Can you work these out from the model? Positions are in its coordinate system, mm. Face numbers are marked on the shaded views. A direction names the side the tool comes from. Coordinates: 2 decimals unless noted, no trailing zeros. Loops run counter-clockwise (first coordinate to the right, second up) from the corner with the lowest first, then second, coordinate; pieces in that order, holes last. Notation, with made-up numbers: M 23.5,20.25 L 54.5,20.25 A29 cw 54.5,46.25 Z; hole C -28,75 d10. An arc over 180 degrees is marked long. Answer as a JSON object with one key per item and string values. Group by question number.
Item 1: Suppose I cut it at A-A (z = -14). Write out the boundary of the cut face in (x, y).
Item 2: Which directions (+Z, -Z, +X, -X, +Y, -Y) give clear straight access to the entire face, cutting with the end or side of a thin tool? Please do the marked faces 1, 2 and 3.
Item 3: If I drill on line 1 (Z direction, x = 0, y = -2.75); line 2 (Y direction, x = 4.25, z = -21); line 3 (X direction, y = -2.5, z = -1.5), over which ranges is the centre line in solid material (lowest first)?
Item 4: Suppose I cut it at C-C (z = -26). Write out the boundary of the cut face in (x, y), then the cut area to 3 significant figures.
Item 5: We'd pull the mould along Z, two halves only. Please class the marked faces 4, 5 and 6: +Z half, -Z half, draft (parallel to the pull), parting line (faces both ways), or undercut.
Item 6: I'm going to push flat-ended pins straight in: pin 1 Ø5.5 at (x, z) = (2, -16) entering from -Y; pin 2 Ø6 at (x, z) = (0.5, -1) entering from -Y; pin 3 Ø1.5 at (x, y) = (-4.5, -2.5) entering from +Z; pin 4 Ø6 at (x, z) = (0, 0) entering from +Y. Where does each tip first touch, or does it pass through?
Item 7: Suppose I cut it at B-B (x = 0). Count the separate pieces of the cut face and the enclosed holes in it, then the cut area to 3 significant figures.
```python
from build123d import *

# Parameters (mm, degrees)
SKETCH1_R           = 0.75
BOSS_EXTRUDE1_DEPTH = 2.25
CUT_EXTRUDE1_DEPTH  = 7
SKETCH3_W           = 6
SKETCH3_H           = 3.5
CUT_EXTRUDE2_DEPTH  = 1
DRAFT1_ANGLE        = 30
DRAFT2_ANGLE        = 30
SKETCH4_R           = 3.9
CUT_EXTRUDE3_DEPTH  = 2
SKETCH5_R           = 4.8
BOSS_EXTRUDE2_DEPTH = 2
CHAMFER1_SIZE       = 1
SKETCH6_R           = 3
CUT_EXTRUDE4_DEPTH  = 3.5
SKETCH7_R           = 1.5
CUT_EXTRUDE5_DEPTH  = 4


with BuildPart() as part:
    # Sketch1 → Boss-Extrude1 (new body, symmetric)
    with BuildSketch(Plane(origin=(0, 0, 0), x_dir=(1, 0, 0), z_dir=(0, 1, 0))):
        with BuildLine():
            Line((-6.470196323, 0.62173913), (-3.732805571, 29.108695652))
            ThreePointArc((-3.732805571, 29.108695652), (0, 32.5), (3.732805571, 29.108695652))
            Line((3.732805571, 29.108695652), (6.470196323, 0.62173913))
            ThreePointArc((6.470196323, 0.62173913), (0, -6.5), (-6.470196323, 0.62173913))
        make_face()
        with Locations((0, 29)):
            Circle(SKETCH1_R, mode=Mode.SUBTRACT)
        with Locations((0, 26)):
            Circle(SKETCH1_R, mode=Mode.SUBTRACT)
        with Locations((0, 23)):
            Circle(SKETCH1_R, mode=Mode.SUBTRACT)
        with Locations((0, 20)):
            Circle(SKETCH1_R, mode=Mode.SUBTRACT)
        with Locations((0, 17)):
            Circle(SKETCH1_R, mode=Mode.SUBTRACT)
        with Locations((0, 14)):
            Circle(SKETCH1_R, mode=Mode.SUBTRACT)
    extrude(amount=BOSS_EXTRUDE1_DEPTH, both=True)

    # Sketch2 → Cut-Extrude1 (cut, symmetric)
    with BuildSketch(Plane(origin=(0, 0, 0), x_dir=(0, 0, -1), z_dir=(1, 0, 0))):
        Polygon((5.5, 2.25), (32.5, 2.25), (32.5, 1.25), (8.5, 1.25), align=None)
    cut_extrude1 = extrude(amount=CUT_EXTRUDE1_DEPTH, both=True, mode=Mode.SUBTRACT)

    # Sketch3 → Cut-Extrude2 (cut)
    with BuildSketch(Plane(origin=(0, 2.25, 0), x_dir=(1, 0, 0), z_dir=(0, 1, 0))):
        with Locations((0, 6.75)):
            Rectangle(SKETCH3_W, SKETCH3_H)
    cut_extrude2 = extrude(amount=-CUT_EXTRUDE2_DEPTH, mode=Mode.SUBTRACT)

    # Mirror1: Cut-Extrude1, Cut-Extrude2 across plane
    add(cut_extrude1.mirror(Plane.ZX), mode=Mode.SUBTRACT)
    add(cut_extrude2.mirror(Plane.ZX), mode=Mode.SUBTRACT)

    # Draft1
    draft1_faces = [part.faces().sort_by_distance(p)[0] for p in [
        (0, 1.75, -5),
        (-3, 1.625, -6.1875),
        (3, 1.625, -6.1875),
    ]]
    draft(draft1_faces, Plane.ZX.offset(2.25), DRAFT1_ANGLE)

    # Draft2
    draft2_faces = [part.faces().sort_by_distance(p)[0] for p in [
        (-3, -1.625, -6.1875),
        (0, -1.75, -5),
        (3, -1.625, -6.1875),
    ]]
    draft(draft2_faces, Plane(origin=(0, -2.25, 0), x_dir=(0, 0, -1), z_dir=(0, -1, 0)), DRAFT2_ANGLE)

    # Sketch4 → Cut-Extrude3 (cut)
    with BuildSketch(Plane(origin=(0, 2.25, 0), x_dir=(1, 0, 0), z_dir=(0, 1, 0))):
        Circle(SKETCH4_R)
    extrude(amount=-CUT_EXTRUDE3_DEPTH, mode=Mode.SUBTRACT)

    # Sketch5 → Boss-Extrude2 (add)
    with BuildSketch(Plane.XZ.offset(2.25)):
        Circle(SKETCH5_R)
    extrude(amount=BOSS_EXTRUDE2_DEPTH)

    # Chamfer1
    chamfer1_edges = [part.edges().sort_by_distance(p)[0] for p in [
        (-4.8, -4.25, 0),
    ]]
    chamfer(chamfer1_edges, length=CHAMFER1_SIZE)

    # Sketch6 → Cut-Extrude4 (cut)
    with BuildSketch(Plane.XZ.offset(4.25)):
        Circle(SKETCH6_R)
    extrude(amount=-CUT_EXTRUDE4_DEPTH, mode=Mode.SUBTRACT)

    # Sketch7 → Cut-Extrude5 (cut, through all)
    with BuildSketch(Plane.XZ.offset(0.75)):
        Circle(SKETCH7_R)
    extrude(amount=-CUT_EXTRUDE5_DEPTH, mode=Mode.SUBTRACT)


solid = part.part
```
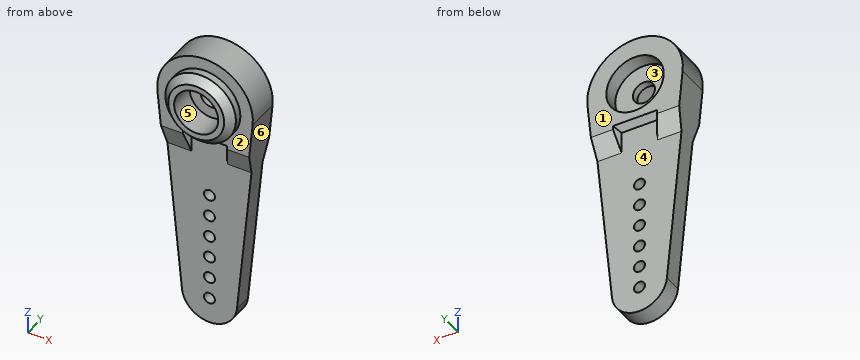
From the geometry:
{
 "1": {"outline": "M -5.18,-1.25 L -0.75,-1.25 L -0.75,1.25 L -5.18,1.25 Z; M 0.75,-1.25 L 5.18,-1.25 L 5.18,1.25 L 0.75,1.25 Z"},
 "2": {"face 1": "+Z, -Z, +X, -X, +Y", "face 2": "-Y", "face 3": "+Y"},
 "3": {"line 1": "-4.8 to -3, 3 to 4.8", "line 2": "-1.25 to 1.25", "line 3": "-4.56 to -2.6, 2.6 to 4.56"},
 "4": {"outline": "M -4.03,-1.25 L -0.75,-1.25 L -0.75,1.25 L -4.03,1.25 Z; M 0.75,-1.25 L 4.03,-1.25 L 4.03,1.25 L 0.75,1.25 Z", "area": "16.4 mm2"},
 "5": {"face 4": "draft", "face 5": "undercut", "face 6": "-Z half"},
 "6": {"pin 1": "y = -1.25", "pin 2": "y = -4.25", "pin 3": "z = 5.28", "pin 4": "y = 0.25"},
 "7": {"separate pieces": "8", "enclosed holes": "0", "area": "77.2 mm2"}
}
